Read the model definition and answer for the solid it produces. Units are mm, in the model's axes. Give positions to 0.01 mm unless a question says otherwise; leave off trailing zeros. Loops run counter-clockwise (first coordinate to the right, second up) from the corner with the lowest first, then second, coordinate; pieces in that order, holes last.
(1) Find section D-D, the plane x = 7. Write down the section's boundary in (y, z).
(2) Find section C-C, the plane y = -74.5. Write down the section's boundary in (x, z).
(3) Find section B-B, the plane z = 49.5. Write down the section's boundary in (x, y).
(4) Find section A-A, the plane z = 87. Write down the section's boundary in (x, y).
(5) Each of these flat-tipped pins is pushed along its axis until it touches: P1, Ø1, axis at x = -55.5, z = 87.5, coming from the -Y side; P2, Ø2.5, axis at x = -78, y = -52, coming from the +Z side; P3, Ø4, axis at x = 60, y = 4, coming from the -Z side; P4, Ø11, axis at y = 5, z = 73, coming from the -X side. Where does it stop, or does it pass through?
(6) Straight lines are drawn through the part: probe 1 along Y at (x, z) = (-60, 89.25); probe 2 along Z at (x, y) = (62.5, 70); probe 3 along X at (y, z) = (44, 24.5). For each, find the intervals that lie inside material, in ascending order.
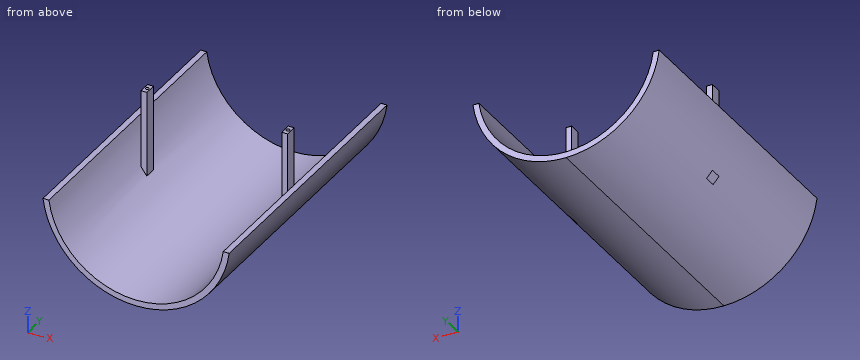
```python
from build123d import *

# Parameters (mm, degrees)
Y_KSEKLIK_EKSTR_ZYON1_DEPTH = 70
IZIM12_W                    = 10
IZIM12_H                    = 70
KES_EKSTR_ZYON11_DEPTH      = 242
IZIM3_W                     = 100
IZIM3_H                     = 10
Y_KSEKLIK_EKSTR_ZYON4_DEPTH = 2.5
KES_EKSTR_ZYON12_START      = -1
KES_EKSTR_ZYON12_DEPTH      = 10
IZIM14_R                    = 1.5
KES_EKSTR_ZYON13_DEPTH      = 27


# Read off the part's stored shape, not the designer's step: Kes-Ekstr_zyon12
with BuildPart() as part:
    # izim1 → Y_kseklik-Ekstr_zyon1 (new body)
    with BuildSketch(Plane.XY):
        with BuildLine():
            Line((-80, 120), (80, 120))
            ThreePointArc((80, 120), (87.071067812, 117.071067812), (90, 110))
            Line((90, 110), (90, -110))
            ThreePointArc((90, -110), (87.071067812, -117.071067812), (80, -120))
            Line((80, -120), (-80, -120))
            ThreePointArc((-80, -120), (-87.071067812, -117.071067812), (-90, -110))
            Line((-90, -110), (-90, 110))
            ThreePointArc((-90, 110), (-87.071067812, 117.071067812), (-80, 120))
        make_face()
    extrude(amount=Y_KSEKLIK_EKSTR_ZYON1_DEPTH)

    # izim12 → Kes-Ekstr_zyon11 (cut)
    with BuildSketch(Plane(origin=(0, 120, 0), x_dir=(1, 0, 0), z_dir=(0, 1, 0))):
        with BuildLine():
            ThreePointArc((-79.372539332, -70), (-52.915026144, -19.999999932), (2.06e-07, 0))
            Line((2.06e-07, 0), (-80, 0))
            Line((-80, 0), (-80, -70))
            Line((-80, -70), (-79.372539332, -70))
        make_face()
        with Locations((-85, -35)):
            Rectangle(IZIM12_W, IZIM12_H)
        with BuildLine():
            Line((-74.330343737, -70), (74.330343737, -70))
            ThreePointArc((74.330343737, -70), (0, -5), (-74.330343737, -70))
        make_face()
        with BuildLine():
            Line((80, -70), (80, 0))
            Line((80, 0), (2.06e-07, 0))
            ThreePointArc((2.06e-07, 0), (52.915026299, -20.000000068), (79.372539332, -70))
            Line((79.372539332, -70), (80, -70))
        make_face()
        with Locations((85, -35)):
            Rectangle(IZIM12_W, IZIM12_H)
    extrude(amount=-KES_EKSTR_ZYON11_DEPTH, mode=Mode.SUBTRACT)

    # izim3 → Y_kseklik-Ekstr_zyon4 (add, symmetric)
    with BuildSketch(Plane(origin=(-60, 0, 0), x_dir=(0, 0, -1), z_dir=(1, 0, 0))):
        with Locations((-55, 4)):
            Rectangle(IZIM3_W, IZIM3_H)
    y_kseklik_ekstr_zyon4 = extrude(amount=Y_KSEKLIK_EKSTR_ZYON4_DEPTH, both=True)

    # Kes-Ekstr_zyon12 outline → Kes-Ekstr_zyon12 (cut)
    with BuildSketch(Plane(origin=(0, 0, 0), x_dir=(1, 0, 0), z_dir=(0, 1, 0)).offset(KES_EKSTR_ZYON12_START)):
        with BuildLine():
            ThreePointArc((-62.5, -30.062539111), (-60.067270979, -27.16134978), (-57.5, -24.378511347))
            Line((-57.5, -24.378511347), (-57.5, -5))
            Line((-57.5, -5), (-62.5, -5))
            Line((-62.5, -5), (-62.5, -30.062539111))
        make_face()
    kes_ekstr_zyon12 = extrude(amount=KES_EKSTR_ZYON12_DEPTH, mode=Mode.SUBTRACT)

    # izim14 → Kes-Ekstr_zyon13 (cut)
    with BuildSketch(Plane.XY.offset(105)):
        with Locations((-60, 4)):
            Circle(IZIM14_R)
    kes_ekstr_zyon13 = extrude(amount=-KES_EKSTR_ZYON13_DEPTH, mode=Mode.SUBTRACT)

    # Aynalama4: Y_kseklik-Ekstr_zyon4, Kes-Ekstr_zyon12, Kes-Ekstr_zyon13 across plane
    add(y_kseklik_ekstr_zyon4.mirror(Plane(origin=(0, 0, 0), x_dir=(0, 0, 1), z_dir=(1, 0, 0))))
    add(kes_ekstr_zyon12.mirror(Plane(origin=(0, 0, 0), x_dir=(0, 0, 1), z_dir=(1, 0, 0))), mode=Mode.SUBTRACT)
    add(kes_ekstr_zyon13.mirror(Plane(origin=(0, 0, 0), x_dir=(0, 0, 1), z_dir=(1, 0, 0))), mode=Mode.SUBTRACT)


solid = part.part
```
Entries:
1. outline: (-120, 0.31) - (120, 0.31) - (120, 5.33) - (-120, 5.33) - close
2. outline: (-79.37, 70) arc R80 ccw to (79.37, 70) - (74.33, 70) arc R75 cw to (-74.33, 70) - close
3. outline: (-73.96, -120) - (-68.52, -120) - (-68.52, 120) - (-73.96, 120) - close; (-62.5, -1) - (-57.5, -1) - (-57.5, 9) - (-62.5, 9) - close; (57.5, -1) - (62.5, -1) - (62.5, 9) - (57.5, 9) - close; (68.52, -120) - (73.96, -120) - (73.96, 120) - (68.52, 120) - close
4. outline: (-62.5, -1) - (-57.5, -1) - (-57.5, 9) - (-62.5, 9) - close; (57.5, -1) - (62.5, -1) - (62.5, 9) - (57.5, 9) - close; hole circle Ø3 at (-60, 4); hole circle Ø3 at (60, 4)
5. P1: passes through
5. P2: stops at z = 70
5. P3: stops at z = 24.9
5. P4: stops at x = -79.37
6. probe 1: y = -1 to 2.5, 5.5 to 9
6. probe 2: z = 30.06 to 38.54
6. probe 3: x = -57.62 to -50.45, 50.45 to 57.62
